from build123d import *

# Parameters (mm, degrees)
ESQUISSE1_R        = 1.5
BOSS_EXTRU_1_DEPTH = 13
CHANFREIN1_SIZE    = 0.25


with BuildPart() as part:
    # Esquisse1 → Boss.-Extru.1 (new body)
    with BuildSketch(Plane.XY):
        Polygon((-1.1875, -2.056810334), (1.1875, -2.056810334), (2.375, 0), (1.1875, 2.056810334), (-1.1875, 2.056810334), (-2.375, 0), align=None)
        with Locations(Location((0, 0, 0), (0, 0, 180))):
            Circle(ESQUISSE1_R, mode=Mode.SUBTRACT)
    extrude(amount=BOSS_EXTRU_1_DEPTH)

    # Chanfrein1
    chanfrein1_edges = [part.edges().sort_by_distance(p)[0] for p in [
        (-1.78125, 1.028405167, 0),
        (0, 2.056810334, 0),
        (1.78125, 1.028405167, 0),
        (1.78125, -1.028405167, 0),
        (0, -2.056810334, 0),
        (-1.78125, -1.028405167, 0),
    ]]
    chamfer(chanfrein1_edges, length=CHANFREIN1_SIZE)


solid = part.part
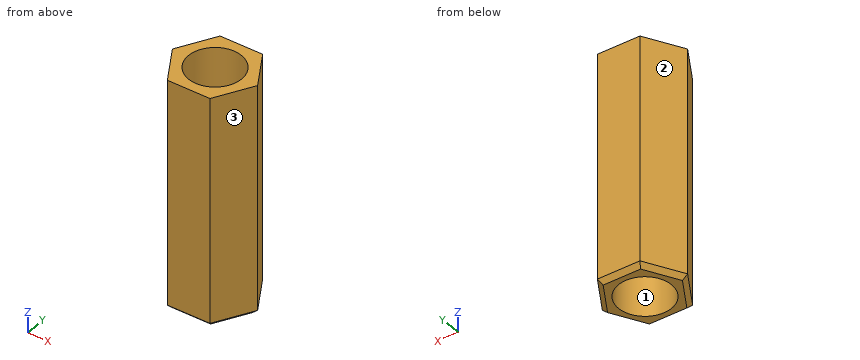
Read the model definition and answer for the solid it produces. Units are mm, in the model's axes. Face numbers are marked on the shaded views. Coordinates: 2 decimals unless noted, no trailing zeros. Order: outer loops, then holes, each group sorted by start corner. A loop starts at its lowest first (then second) coordinate and runs counter-clockwise, first axis right, second up. Notation, with made-up numbers: M 72.5,47.5 L 112.5,47.5 A20 cw 112.5,70.5 Z; hole C -7,68 d7. An arc over 180 degrees is marked long. Put each result on its own line as item: value. Start each with the question number.
Item 1: Section D-D, the plane x = -1.65 is taken. Determine the outline of the cut face in (y, z), plus the area to 3 significant figures.
Item 2: Consider probe 1 along Y at (x, z) = (0, 10.5); probe 2 along X at (y, z) = (-0.8, 7.5); probe 3 along Y at (x, z) = (-0.55, 5.75). Determine where each line is inside the solid, lowest interval first. Write a range as [from, to].
Item 3: Section C-C, the plane y = 0.65 is taken. Determine the outline of the cut face in (x, z).
Item 4: Section A-A, the plane z = 1 is taken. Determine the outline of the cut face in (x, y) (1 decimal), plus the area to 3 significant figures.
Item 5: Given pin 1 Ø1.5 at (x, y) = (-2, -1) entering from -Z, flat-ended and moving along its own axis, determine where the tip first touches the part or whether it passes through.
Item 6: The mould has two halves that part along Y. Classify the marked faces 1, 2 and 3: +Y half, -Y half, draft (parallel to the pull), parting line (faces both ways), or undercut.
Item 7: Section B-B, the plane x = -0.5 is taken. Determine the outline of the cut face in (y, z), plus the area to 3 significant figures.
Computed:
1. outline: M -1.26,0.25 L -0.76,0 L 0.76,0 L 1.26,0.25 L 1.26,13 L -1.26,13 Z
1. area: 32.5 mm2
2. probe 1: y = [-2.06, -1.5], [1.5, 2.06]
2. probe 2: x = [-1.91, -1.27], [1.27, 1.91]
2. probe 3: y = [-2.06, -1.4], [1.4, 2.06]
3. outline: M -2,0.25 L -1.71,0 L -1.35,0 L -1.35,13 L -2,13 Z; M 1.35,0 L 1.71,0 L 2,0.25 L 2,13 L 1.35,13 Z
4. outline: M -2.4,0 L -1.2,-2.1 L 1.2,-2.1 L 2.4,0 L 1.2,2.1 L -1.2,2.1 Z; hole C 0,0 d3
4. area: 7.59 mm2
5. pin 1: stops at z = 0
6. face 1: undercut
6. face 2: +Y half
6. face 3: -Y half
7. outline: M -2.06,0.25 L -1.81,0 L -1.41,0 L -1.41,13 L -2.06,13 Z; M 1.41,0 L 1.81,0 L 2.06,0.25 L 2.06,13 L 1.41,13 Z
7. area: 16.6 mm2
